```python
from build123d import *

# Parameters (mm, degrees)
F0_W     = 203.2
F0_H     = 127
F1_DEPTH = 127
F3_DEPTH = 76.2
F4_SIZE2 = 101.6
F4_SIZE  = 76.2
F5_R     = 5.08
F6_R     = 15.24
F7_DEPTH = 50.8
F8_R     = 12.7
F9_DEPTH = 127


with BuildPart() as f1:
    # F0 (on Front) → F1 (new body)
    with BuildSketch(Plane.XZ):
        with Locations((-34.4487503171, -10.7558194239)):
            Rectangle(F0_W, F0_H)
    extrude(amount=F1_DEPTH)

    # F2 (on face) → F3 (cut)
    with BuildSketch(Plane.XZ.offset(127)):
        Polygon((67.1512496829, 52.7441805761), (-34.4487503171, 52.7441805761), (-34.4487503171, -10.7558194239), (-72.5487503171, -10.7558194239), (-72.5487503171, -74.2558194239), (67.1512496829, -74.2558194239), align=None)
    extrude(amount=-F3_DEPTH, mode=Mode.SUBTRACT)

    # F4
    f4_edges = [f1.edges().sort_by_distance(p)[0] for p in [
        (67.15125, -25.4, 52.744181),
    ]]
    f4_side = f1.faces().sort_by_distance((-56.220179, -52.614286, 52.744181))[0]
    chamfer(f4_edges, length=F4_SIZE, length2=F4_SIZE2, reference=f4_side)

    # F5
    f5_edges = [f1.edges().sort_by_distance(p)[0] for p in [
        (-136.04875, -63.5, 52.744181),
        (-85.24875, -127, 52.744181),
        (-34.44875, -127, 20.994181),
        (-53.49875, -127, -10.755819),
        (-72.54875, -127, -42.505819),
        (-72.54875, -50.8, -42.505819),
        (-34.44875, -88.9, -10.755819),
        (-34.44875, -88.9, 52.744181),
        (-21.74875, -50.8, 52.744181),
        (-72.54875, 0, 52.744181),
        (-9.04875, -25.4, 52.744181),
    ]]
    fillet(f5_edges, radius=F5_R)

    # F6 (on face) → F7 (cut, through all)
    with BuildSketch(Plane.XZ.offset(50.8)):
        with Locations((-16.6687503171, -28.5358194239)):
            Circle(F6_R)
    extrude(amount=-F7_DEPTH, mode=Mode.SUBTRACT)

    # F8 (on face) → F9 (cut, through all)
    with BuildSketch(Plane.XY.offset(52.7441805761)):
        with Locations((-90.3287503171, -68.58)):
            Circle(F8_R)
    extrude(amount=-F9_DEPTH, mode=Mode.SUBTRACT)


solid = f1.part
```
Read the model definition and answer for the solid it produces. Units are mm, in the model's axes. A direction names the side the tool comes from. Give positions to 0.01 mm unless a question says otherwise; leave off trailing zeros. Write each loop counter-clockwise with the first axis right and the second up, starting at its lowest first coordinate (ties: lowest second). Pieces come first, ordered by that corner, then holes. Notation, with made-up numbers: M 65.25,45.5 L 85.25,45.5 A30 ccw 85.25,78.5 Z; hole C 58.25,44 d11. An arc over 180 degrees is marked long. Put each result on its own line as item: value. Start each with the question number.
1. The part is cut by section A-A, the plane y = -68.58. Give the vertices of the cut face in (x, z), and give its area (3 significant figures).
2. The part is cut by section C-C, the plane x = -97.5. Give the vertices of the cut face in (y, z).
3. The part is cut by section D-D, the plane z = -46. Give the vertices of the cut face in (x, y).
4. For a pull along Y with two mould halves and no side action, classify faces 1 (the flat face through (67.151, -25, -62)), 2 (the cylindrical face through (-74.076, -125.551, -40.446)), 3 (the cylindrical face through (-78.597, -73.444, -9.867)), 4 (the cylindrical face through (-69.73, -1.53, 51.3)) as released by +Y, released by -Y, zero draft, split by the parting line, or undercut.
5. The part is cut by section B-B, the plane y = -94. Give the vertices of the cut face in (x, z).
6. Consider line 1 along Y through (x, z) = (13, -63.5); line 2 along X through (y, z) = (-51.5, 40); line 3 along X through (y, z) = (-73.5, 18.5). Determine where each line is inside the solid, lowest interval first.
7. Which of the six approach directions +Z, -Z, +X, -X, +Y, -Y give full straight-line access (tool end or side, diameter ignored) to faces 5 (the flat face through (-56, -87, -10.756)), 6 (the cylindrical face through (-35.98, -83.29, 51.3)), 7 (the flat face through (-72, -63, 52.744))?
8. Each of these flat-tipped pins is pushed along its axis until it touches: pin 1 Ø2 at (x, z) = (28.5, -43.5) entering from +Y; pin 2 Ø4 at (x, z) = (-27.5, -14) entering from -Y; pin 3 Ø10 at (y, z) = (-22, -22) entering from +X; pin 4 Ø10 at (y, z) = (-45.5, 3.5) entering from +X. Where does it stop, or does it pass through?
Final values:
1. outline: M -136.05,-74.26 L -103.03,-74.26 L -103.03,52.74 L -130.97,52.74 A5.08 ccw -136.05,47.66 Z; M -77.63,-74.26 L -72.55,-74.26 L -72.55,-10.76 L -39.53,-10.76 A5.08 ccw -34.45,-5.68 L -34.45,47.66 A5.08 ccw -39.53,52.74 L -77.63,52.74 Z
1. area: 7,240 mm²
2. outline: M -127,-74.26 L -79.06,-74.26 L -79.06,52.74 L -121.92,52.74 A5.08 ccw -127,47.66 Z; M -58.1,-74.26 L 0,-74.26 L 0,47.66 A5.08 ccw -5.08,52.74 L -58.1,52.74 Z
3. outline: M -136.05,-127 L -77.63,-127 A5.08 ccw -72.55,-121.92 L -72.55,-55.88 A5.08 cw -67.47,-50.8 L 65.01,-50.8 L 65.01,0 L -136.05,0 Z; hole C -90.33,-68.58 d25.4
4. face 1: zero draft
4. face 2: released by -Y
4. face 3: undercut
4. face 4: released by +Y
5. outline: M -136.05,-74.26 L -72.55,-74.26 L -72.55,-10.76 L -39.53,-10.76 A5.08 ccw -34.45,-5.68 L -34.45,47.66 A5.08 ccw -39.53,52.74 L -130.97,52.74 A5.08 ccw -136.05,47.66 Z
6. line 1: y = -50.8 to 0
6. line 2: x = -136.05 to -34.45
6. line 3: x = -136.05 to -102.04, -78.62 to -34.45
7. face 5: -Z, +X, -Y
7. face 6: +Z, +X, -Y
7. face 7: +Z, +X, -X, +Y, -Y
8. pin 1: stops at y = 0
8. pin 2: stops at y = -50.8
8. pin 3: stops at x = 50.76
8. pin 4: stops at x = 31.63
